Autodesk Inventor part; units mm, degrees
ref_plane "YZ Plane" through (0, 0, 0) normal (1, 0, 0) x (0, 1, 0)
ref_plane "XZ Plane" through (0, 0, 0) normal (0, 1, 0) x (-1, 0, 0)
ref_plane "XY Plane" through (0, 0, 0) normal (0, 0, 1) x (1, 0, 0)
sketch "Sketch1" plane through (0, 0, 0) normal (0, 0, 1) x (1, 0, 0)
  line L0 (-13.25, 14.85) -> (13.25, 14.85)
  line L1 (13.25, 14.85) -> (13.25, -14.85)
  line L2 (13.25, -14.85) -> (-13.25, -14.85)
  line L3 (-13.25, -14.85) -> (-13.25, 14.85)
  line L4 (-13.25, 14.85) -> (13.25, -14.85) construction
  line L5 (13.25, 14.85) -> (-13.25, -14.85) construction
  point P0 (0, 0)
  dimension "d0" = 26.5
  dimension "d1" = 29.7
extrude "Extrusion1" add sketch "Sketch1" along normal blind 8.5
sketch "Sketch2" plane through (0, 0, 8.5) normal (0, 0, 1) x (1, 0, 0)
  line L0 (-8.8, 6.85) -> (8.8, 6.85)
  line L1 (8.8, 6.85) -> (8.8, -6.85)
  line L2 (8.8, -6.85) -> (-8.8, -6.85)
  line L3 (-8.8, -6.85) -> (-8.8, 6.85)
  line L4 (-8.8, 6.85) -> (8.8, -6.85) construction
  line L5 (8.8, 6.85) -> (-8.8, -6.85) construction
  point P0 (0, 0)
  dimension "d4" = 17.6
  dimension "d5" = 13.7
extrude "Extrusion2" add sketch "Sketch2" along normal blind 5
fillet "Fillet1" radius 6.8 4 edges at (8.8, 6.85, 11) (8.8, -6.85, 11) (-8.8, 6.85, 11) (-8.8, -6.85, 11)
sketch "Sketch3" plane through (0, 0, 13.5) normal (0, 0, 1) x (1, 0, 0)
  circle A0 centre (0, 0) radius 6.825
  dimension "d9" = 13.65
extrude "Extrusion3" add sketch "Sketch3" along normal blind 5
sketch "Sketch4" plane through (0, 0, 18.5) normal (0, 0, 1) x (1, 0, 0)
  circle A0 centre (0, 0) radius 3
  dimension "d12" = 6
extrude "Extrusion4" add sketch "Sketch4" along normal blind 11
sketch "Sketch5" plane through (0, 0, 0) normal (0, 0, -1) x (-1, 0, 0)
  line L0 (-10, 12.5) -> (10, 12.5) construction
  line L1 (10, 12.5) -> (10, -12.5) construction
  line L2 (10, -12.5) -> (-10, -12.5) construction
  line L3 (-10, -12.5) -> (-10, 12.5) construction
  line L4 (-10, 12.5) -> (10, -12.5) construction
  line L5 (10, 12.5) -> (-10, -12.5) construction
  circle A0 centre (10, 12.5) radius 0.4
  circle A1 centre (-10, -12.5) radius 0.4
  circle A2 centre (10, -12.5) radius 0.4
  circle A3 centre (-10, 12.5) radius 0.4
  point P0 (0, 0)
  dimension "d15" = 20
  dimension "d16" = 25
  dimension "d18" = 0.8
  dimension "d19" = 0.8
  dimension "d20" = 0.8
  dimension "d21" = 0.8
extrude "Extrusion5" add sketch "Sketch5" along normal blind 3
sketch "Sketch6" plane through (0, 0, 0) normal (0, 0, -1) x (-1, 0, 0)
  circle A0 centre (0, 0) radius 6.825
extrude "Extrusion6" add sketch "Sketch6" along normal blind 4
properties part number "Encoder" material "ABS Plastic"
Source: CAD feature listing. Evaluate the final solid. Frame: model axes, mm. A direction names the side the tool comes from. Give positions to 0.01 mm unless a question says otherwise; leave off trailing zeros. Order: outer loops, then holes, each group sorted by start corner. A loop starts at its lowest first (then second) coordinate and runs counter-clockwise, first axis right, second up. Notation, with made-up numbers: (56, 2) -> (74, 2) arc R20 ccw to (74, 33) -> close; hole circle Ø3 at (18, 6). An arc over 180 degrees is marked (long way). Use a Markdown table: item, result.
1) Section query D-D, the plane x = -6.25. Return the cut outline in (y, z), then the cut area to 3 significant figures.
Answer list:
| item | result |
|---|---|
| outline | (-14.85, 0) -> (-2.74, 0) -> (-2.74, -4) -> (2.74, -4) -> (2.74, 0) -> (14.85, 0) -> (14.85, 8.5) -> (5.36, 8.5) -> (5.36, 13.5) -> (2.74, 13.5) -> (2.74, 18.5) -> (-2.74, 18.5) -> (-2.74, 13.5) -> (-5.36, 13.5) -> (-5.36, 8.5) -> (-14.85, 8.5) -> close |
| area | 355 mm² |
2) Section query C-C, the plane y = -1.25. Return the cut outline in (x, z).
Answer list:
| item | result |
|---|---|
| outline | (-13.25, 0) -> (-6.71, 0) -> (-6.71, -4) -> (6.71, -4) -> (6.71, 0) -> (13.25, 0) -> (13.25, 8.5) -> (8.69, 8.5) -> (8.69, 13.5) -> (6.71, 13.5) -> (6.71, 18.5) -> (2.73, 18.5) -> (2.73, 29.5) -> (-2.73, 29.5) -> (-2.73, 18.5) -> (-6.71, 18.5) -> (-6.71, 13.5) -> (-8.69, 13.5) -> (-8.69, 8.5) -> (-13.25, 8.5) -> close |
3) Reachability of faces 4 (the cylindrical face through (-10.185, -12.145, -1.479)), 5 (the cylindrical face through (6.861, 4.805, 11.035)), 6 (the cylindrical face through (-6.861, -4.805, 11.035)) from +Z, -Z, +X, -X, +Y, -Y: full face, straight path, thin tool, end or side. Return the list, or none.
Answer list:
| item | result |
|---|---|
| face 4 | -Z |
| face 5 | +Z, +X, +Y |
| face 6 | +Z, -X, -Y |
4) Contact query for flat-ended pins moving along their axis: P1, Ø3, axis at x = -6.5, z = 10.5, coming from the -Y side; P2, Ø11, axis at x = 2.5, y = 3, coming from the +Z side; P3, Ø5, axis at x = -8, y = -5.5, coming from the +Z side; P4, Ø4.5, axis at x = 0.5, z = 11.5, coming from the +Y side. Output: stop coordinate, or through.
Answer list:
| item | result |
|---|---|
| P1 | y = -6.15 |
| P2 | z = 29.5 |
| P3 | z = 13.5 |
| P4 | y = 6.85 |
5) Mould query, pull axis X, two halves, no side actions, for faces 1 (the cylindrical face through (-3, 0, 24)), 2 (the flat face through (10, -12.5, -3)), 3 (the cylindrical face through (9.815, 12.855, -1.479)). Classes: +X half, -X half, draft (parallel to the pull), parting line (faces both ways), or undercut.
Answer list:
| item | result |
|---|---|
| face 1 | parting line |
| face 2 | draft |
| face 3 | undercut |
6) Section query B-B, the plane z = 13. Return the cut outline in (x, y), then the cut area to 3 significant figures.
Answer list:
| item | result |
|---|---|
| outline | (-8.8, -0.05) arc R6.8 ccw to (-2, -6.85) -> (2, -6.85) arc R6.8 ccw to (8.8, -0.05) -> (8.8, 0.05) arc R6.8 ccw to (2, 6.85) -> (-2, 6.85) arc R6.8 ccw to (-8.8, 0.05) -> close |
| area | 201 mm² |
7) Section query A-A, the plane x = 0. Return the cut outline in (y, z) (3 decimals).
Answer list:
| item | result |
|---|---|
| outline | (-14.85, 0) -> (-6.825, 0) -> (-6.825, -4) -> (6.825, -4) -> (6.825, 0) -> (14.85, 0) -> (14.85, 8.5) -> (6.85, 8.5) -> (6.85, 13.5) -> (6.825, 13.5) -> (6.825, 18.5) -> (3, 18.5) -> (3, 29.5) -> (-3, 29.5) -> (-3, 18.5) -> (-6.825, 18.5) -> (-6.825, 13.5) -> (-6.85, 13.5) -> (-6.85, 8.5) -> (-14.85, 8.5) -> close |
8) Ray query, line 1 along Z through (x, y) = (3.5, -6.5); line 2 along Z through (x, y) = (12.25, 1); line 3 along X through (y, z) = (0.25, 22). Return the intervals inside material, ascending. Write a range as [from, to].
Answer list:
| item | result |
|---|---|
| line 1 | [0, 13.5] |
| line 2 | [0, 8.5] |
| line 3 | [-2.99, 2.99] |
